from build123d import *

# Parameters (mm, degrees)
BOSS_EXTRUDE1_REACH      = 596.549
BOSS_EXTRUDE1_END_RADIUS = 25
SKETCH3_W                = 47.52
SKETCH3_H                = 16


with BuildPart() as part:
    # Sketch1 → Revolve1 (revolve)
    with BuildSketch(Plane.XY):
        Polygon((-588.665, 0), (-588.665, 25), (-541.145, 25), (-541.145, 42.5), (541.145, 42.5), (541.145, 25), (588.665, 25), (588.665, 0), align=None)
    revolve(axis=Axis((588.665, 0, 0), (-1, 0, 0)))

    # Boss-Extrude1: up to this cylinder (the profile starts outside it)
    boss_extrude1_end = Plane(origin=(0, 0, 0), z_dir=(1, 0, 0)) * Cylinder(BOSS_EXTRUDE1_END_RADIUS, 2373.908, mode=Mode.PRIVATE)
    # Sketch3 → Boss-Extrude1 (add, up to the surface)
    with BuildSketch(Plane.XY.offset(29.3), mode=Mode.PRIVATE) as boss_extrude1_sk1:
        with Locations((-564.905, 0)):
            Rectangle(SKETCH3_W, SKETCH3_H)
    boss_extrude1_tool1 = extrude(boss_extrude1_sk1.sketch, amount=-BOSS_EXTRUDE1_REACH, mode=Mode.PRIVATE) - boss_extrude1_end
    add(boss_extrude1_tool1.solids().sort_by_distance((-564.905, 0, 29.3))[0])
    # Sketch3 → Boss-Extrude1 (add, up to the surface)
    with BuildSketch(Plane.XY.offset(29.3), mode=Mode.PRIVATE) as boss_extrude1_sk2:
        with Locations((564.905, 0)):
            Rectangle(SKETCH3_W, SKETCH3_H)
    boss_extrude1_tool2 = extrude(boss_extrude1_sk2.sketch, amount=-BOSS_EXTRUDE1_REACH, mode=Mode.PRIVATE) - boss_extrude1_end
    add(boss_extrude1_tool2.solids().sort_by_distance((564.905, 0, 29.3))[0])


solid = part.part
Geometry: final body of the model. Coordinates: model frame, mm. A direction names the side the tool comes from. Round coordinates to 2 decimals unless told otherwise and drop trailing zeros. Loops run counter-clockwise (first coordinate to the right, second up) from the corner with the lowest first, then second, coordinate; pieces in that order, holes last. Notation, with made-up numbers: M 10,85.25 L 31,85.25 A11 cw 31,102.25 Z; hole C 29,54.5 d3. An arc over 180 degrees is marked long. Put each result on its own line as item: value. Start each with the question number.
(1) Material intervals for line 1 along X through (y, z) = (34.5, -5.5) (3 decimals); line 2 along Y through (x, z) = (-463, 2.5); line 3 along Z through (x, y) = (423, -4), sorted ascending. Write a range as [from, to].
(2) Section query A-A (z = 0). Return loops of the section in (x, y) (3 decimals).
(3) Contact query for flat-ended pins moving along their axis: pin 1 Ø4 at (x, y) = (168, 21) entering from +Z; pin 2 Ø4.5 at (x, z) = (559.5, 28) entering from +Y; pin 3 Ø1 at (x, z) = (-204.5, -22) entering from -Y. Output: stop coordinate, or through.
(4) Section query B-B (x = -417.5). Return loops of the section in (y, z).
(5) Set-up query: faces 1 (the face through (565.24, 0.99, -24.98)), 2 (the face through (-564.57, 0.99, -24.98)), 3 (the face through (-588.665, 0, 2)). Return all of +Z, -Z, +X, -X, +Y, -Y with unobstructed straight access to the full face (end or side cutting, diameter ignored); none if empty.
Findings below:
1. line 1: x = [-541.145, 541.145]
1. line 2: y = [-42.43, 42.43]
1. line 3: z = [-42.31, 42.31]
2. outline: M -588.665,-25 L -541.145,-25 L -541.145,-42.5 L 541.145,-42.5 L 541.145,-25 L 588.665,-25 L 588.665,25 L 541.145,25 L 541.145,42.5 L -541.145,42.5 L -541.145,25 L -588.665,25 Z
3. pin 1: stops at z = 38.02
3. pin 2: stops at y = 8
3. pin 3: stops at y = -36.66
4. outline: C 0,0 d85
5. face 1: +X
5. face 2: -X
5. face 3: +Z, -Z, -X, +Y, -Y
